Design review of the part built by this model. Coordinates are the model's own, in mm. A direction names the side the tool comes from. Give positions to 0.01 mm unless a question says otherwise; leave off trailing zeros. Write each loop counter-clockwise with the first axis right and the second up, starting at its lowest first coordinate (ties: lowest second). Pieces come first, ordered by that corner, then holes. Notation, with made-up numbers: M 1,-14.5 L 47,-14.5 A19 ccw 47,-5.5 Z; hole C 82,77 d1. An arc over 180 degrees is marked long. One line per item, written item: value. Start each with the question number.
```python
from build123d import *

# Parameters (mm, degrees)
F0_W      = 50
F0_H      = 35
F1_DEPTH  = 8
F2_W      = 38
F2_H      = 24
F3_DEPTH  = 4
F4_R      = 3.5
F6_DEPTH  = 2
F5_R      = 3.5
F7_DEPTH  = 2
F8_W      = 6
F8_H      = 5
F9_DEPTH  = 1.5
F10_W     = 50
F10_H     = 3.4
F14_DEPTH = 2.5
F11_W     = 3.4
F11_H     = 35
F15_DEPTH = 2.5
F12_W     = 50
F12_H     = 3.4
F16_DEPTH = 2.5
F13_W     = 3.4
F13_H     = 35
F17_DEPTH = 2.5
F18_R     = 5
F19_R     = 1
F20_R     = 2


with BuildPart() as f1:
    # F0 (on Front) → F1 (new body)
    with BuildSketch(Plane.XZ):
        with Locations((25, 17.5)):
            Rectangle(F0_W, F0_H)
    extrude(amount=F1_DEPTH)

    # F2 (on face) → F3 (cut)
    with BuildSketch(Plane.XZ.offset(8)):
        with Locations((25, 17.5)):
            Rectangle(F2_W, F2_H)
    extrude(amount=-F3_DEPTH, mode=Mode.SUBTRACT)

    # F4 (on face) → F6 (join)
    with BuildSketch(Plane.XZ.offset(4)):
        with Locations((28, 9.5)):
            Circle(F4_R)
    extrude(amount=F6_DEPTH)

    # F5 (on face) → F7 (join)
    with BuildSketch(Plane.XZ.offset(4)):
        with Locations((28, 25.5)):
            Circle(F5_R)
    extrude(amount=F7_DEPTH)

    # F8 (on face) → F9 (cut)
    with BuildSketch(Plane.XZ.offset(8)):
        with Locations((47, 17.5)):
            Rectangle(F8_W, F8_H)
    extrude(amount=-F9_DEPTH, mode=Mode.SUBTRACT)

    # F10 (on face) → F14 (cut)
    with BuildSketch(Plane(origin=(0, 0, 0), x_dir=(1, 0, 0), z_dir=(0, 0, -1))):
        with Locations((25, 4)):
            Rectangle(F10_W, F10_H)
    extrude(amount=-F14_DEPTH, mode=Mode.SUBTRACT)

    # F11 (on face) → F15 (cut)
    with BuildSketch(Plane(origin=(0, 0, 0), x_dir=(0, -1, 0), z_dir=(-1, 0, 0))):
        with Locations((4, 17.5)):
            Rectangle(F11_W, F11_H)
    extrude(amount=-F15_DEPTH, mode=Mode.SUBTRACT)

    # F12 (on face) → F16 (cut)
    with BuildSketch(Plane.XY.offset(35)):
        with Locations((25, -4)):
            Rectangle(F12_W, F12_H)
    extrude(amount=-F16_DEPTH, mode=Mode.SUBTRACT)

    # F13 (on face) → F17 (cut)
    with BuildSketch(Plane.YZ.offset(50)):
        with Locations((-4, 17.5)):
            Rectangle(F13_W, F13_H)
    extrude(amount=-F17_DEPTH, mode=Mode.SUBTRACT)

    # F18
    f18_edges = [f1.edges().sort_by_distance(p)[0] for p in [
        (0, -1.15, 35),
        (0, -6.85, 35),
        (0, -1.15, 0),
        (0, -6.85, 0),
        (50, -1.15, 0),
        (50, -6.85, 0),
        (50, -1.15, 35),
        (50, -6.85, 35),
        (44, -6, 29.5),
        (44, -6, 5.5),
        (6, -6, 5.5),
        (6, -6, 29.5),
    ]]
    fillet(f18_edges, radius=F18_R)

    # F19
    f19_edges = [f1.edges().sort_by_distance(p)[0] for p in [
        (25, -8, 0),
    ]]
    fillet(f19_edges, radius=F19_R)

    # F20
    f20_edges = [f1.edges().sort_by_distance(p)[0] for p in [
        (2.5, -4, 32.5),
        (2.5, -4, 2.5),
        (47.5, -4, 2.5),
        (47.5, -4, 32.5),
    ]]
    fillet(f20_edges, radius=F20_R)


solid = f1.part
```
Q1. For P1, Ø2, axis at x = 28.5, z = 10, coming from the -Y side; P2, Ø1.6, axis at x = 47.5, y = -7.5, coming from the +Z side; P3, Ø1, axis at x = 32, y = -4, coming from the +Z side, all flat-tipped, find the tip position at first contact; note any pin that passes through.
Q2. Take a section at C-C, the plane x = 28. Give the boundary of the cut face in (y, z), then the cut area to 3 significant figures.
Q3. Take a section at A-A, the plane x = 36. Give the boundary of the cut face in (y, z).
Q4. Machinability: for faces 1 (the face through (29.88, -4.99, 28.45)), 2 (the face through (25, -4, 2.5)), 3 (the face through (25, -4, 32.5)), 4 (the face through (25, -2.3, 33)), which of the approach directions +Z, -Z, +X, -X, +Y, -Y give a long, thin tool a straight path to every point of the face, cutting with its end or side? Answer none if there is none.
Q5. Wall thickness on line 1 (Y direction, x = 23, z = 33); line 2 (Y direction, x = 48, z = 19); line 3 (X direction, y = -5.25, z = 24): over which ranges is each line inside the solid? List them lowest first. Write a range as from..to.
Q6. Take a section at D-D, the plane z = 12. Give the boundary of the cut face in (x, y).
Q7. Take a section at B-B, the plane z = 23.5. Give the boundary of the cut face in (x, y).
Q8. The part is to be moulded in two halves that separate along X. For faces 5 (the face through (25, -5.7, 2)), 6 (the face through (1, -6, 33)), 7 (the face through (28, -6, 26)), say which applies: pulls with the +X half, pulls with the -X half, needs draft (parallel to the pull), parting line crosses it, or undercut.
Results list:
1. P1: stops at y = -6
1. P2: stops at z = 34.66
1. P3: stops at z = 32.5
2. outline: M -8,1 A1 ccw -7,0 L -5.7,0 L -5.7,2.5 L -2.3,2.5 L -2.3,0 L 0,0 L 0,35 L -2.3,35 L -2.3,32.5 L -5.7,32.5 L -5.7,35 L -7,35 A1 ccw -8,34 L -8,29.5 L -4,29.5 L -4,29 L -6,29 L -6,22 L -4,22 L -4,13 L -6,13 L -6,6 L -4,6 L -4,5.5 L -8,5.5 Z
2. area: 195 mm^2
3. outline: M -8,1 A1 ccw -7,0 L -5.7,0 L -5.7,2.5 L -2.3,2.5 L -2.3,0 L 0,0 L 0,35 L -2.3,35 L -2.3,32.5 L -5.7,32.5 L -5.7,35 L -7,35 A1 ccw -8,34 L -8,29.5 L -4,29.5 L -4,5.5 L -8,5.5 Z
4. face 1: -Y
4. face 2: -Z, +X, -X
4. face 3: +Z, +X, -X
4. face 4: none
5. line 1: y = -8..-5.7, -2.3..0
5. line 2: y = -6.5..-5.7, -2.3..0
5. line 3: x = 2.5..6, 24.84..31.16, 44..47.5
6. outline: M 0,-7 A1 ccw 1,-8 L 6,-8 L 6,-4 L 25.55,-4 L 25.55,-6 L 30.45,-6 L 30.45,-4 L 44,-4 L 44,-8 L 49,-8 A1 ccw 50,-7 L 50,-5.7 L 47.5,-5.7 L 47.5,-2.3 L 50,-2.3 L 50,0 L 0,0 L 0,-2.3 L 2.5,-2.3 L 2.5,-5.7 L 0,-5.7 Z
7. outline: M 0,-7 A1 ccw 1,-8 L 6,-8 L 6,-4 L 25.13,-4 L 25.13,-6 L 30.87,-6 L 30.87,-4 L 44,-4 L 44,-8 L 49,-8 A1 ccw 50,-7 L 50,-5.7 L 47.5,-5.7 L 47.5,-2.3 L 50,-2.3 L 50,0 L 0,0 L 0,-2.3 L 2.5,-2.3 L 2.5,-5.7 L 0,-5.7 Z
8. face 5: needs draft
8. face 6: pulls with the -X half
8. face 7: undercut
